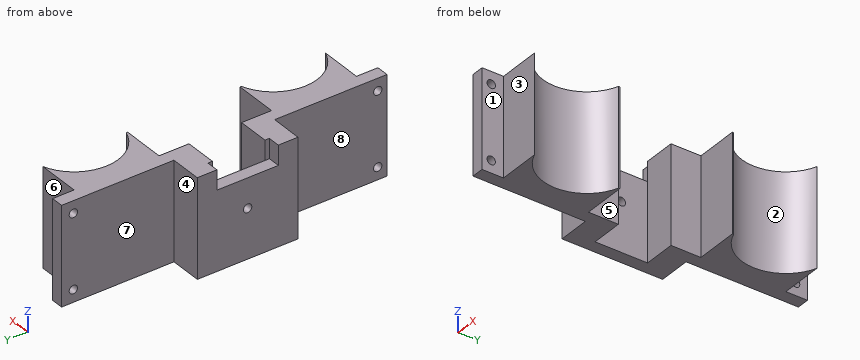
```python
from build123d import *

# Parameters (mm, degrees)
BOSS_EXTRUDE1_DEPTH  = 40
M3_CLEARANCE_HOLE1_D = 3.4
SKETCH6_W            = 5
SKETCH6_H            = 25
CUT_EXTRUDE1_DEPTH   = 8
M3_CLEARANCE_HOLE2_D = 3.4


with BuildPart() as part:
    # Sketch1 → Boss-Extrude1 (new body)
    with BuildSketch(Plane.XY):
        with BuildLine():
            Line((5, 0), (0, 0))
            Line((0, 0), (0, -20.5))
            Line((0, -20.5), (13, -20.5))
            Line((13, -20.5), (13, -66.25))
            Line((13, -66.25), (18, -66.25))
            Line((18, -66.25), (18, -57.5))
            Line((18, -57.5), (35.314368035, -57.5))
            ThreePointArc((35.314368035, -57.5), (23.250292021, -40.40428558), (35.508342613, -23.447116675))
            Line((35.508342613, -23.447116675), (35.508342613, -22.9))
            Line((35.508342613, -22.9), (18, -22.9))
            Line((18, -22.9), (18, -10.7))
            Line((18, -10.7), (5, -10.7))
            Line((5, -10.7), (5, 0))
        make_face()
    boss_extrude1 = extrude(amount=BOSS_EXTRUDE1_DEPTH)

    # Mirror1: Boss-Extrude1 across plane
    add(boss_extrude1.mirror(Plane.ZX))

    # M3 Clearance Hole1 (through all)
    with Locations(Plane.ZY.offset(-13)):
        with Locations((35, -62.481816862), (5, -62.481816862), (35, 61.468183138), (5, 61.468183138)):
            Hole(M3_CLEARANCE_HOLE1_D / 2)

    # Sketch6 → Cut-Extrude1 (cut)
    with BuildSketch(Plane(origin=(0, 0, 40), x_dir=(-1, 0, 0), z_dir=(0, 0, -1))):
        with Locations((-2.5, 0)):
            Rectangle(SKETCH6_W, SKETCH6_H)
    extrude(amount=CUT_EXTRUDE1_DEPTH, mode=Mode.SUBTRACT)

    # M3 Clearance Hole2 (through all)
    with Locations(Plane.ZY):
        with Locations((20, 0)):
            Hole(M3_CLEARANCE_HOLE2_D / 2)


solid = part.part
```
Can you work these out from the model? Positions are in its coordinate system, mm. Face numbers are marked on the shaded views. A direction names the side the tool comes from. Coordinates: 2 decimals unless noted, no trailing zeros. Loops run counter-clockwise (first coordinate to the right, second up) from the corner with the lowest first, then second, coordinate; pieces in that order, holes last. Notation, with made-up numbers: (-29, -3) - (-19, -3) arc R24 ccw to (-19, 31) - close; hole circle Ø2 at (4.5, 78). An arc over 180 degrees is marked (long way). Answer as CSV lines item,"result". Start each with the question number.
1) Thinking about a two-plate mould opening in Y: for the marked faces 1, 2, 3 and 4, which applies, pulls with the +Y half, pulls with the -Y half, needs draft (parallel to the pull), parting line crosses it, or undercut?
2) Suppose I cut it at C-C (x = 16). Please give me the cut outline in (y, z).
3) Which directions (+Z, -Z, +X, -X, +Y, -Y) give clear straight access to the entire face, cutting with the end or side of a thin tool? Please do the marked faces 5, 6, 7 and 8.
4) For pin 1 (1 mm diameter, centred on x = 30.5, z = 29.5, fed in from +Y); pin 2 (7 mm diameter, centred on y = -61.5, z = 19.5, fed in from +X); pin 3 (5 mm diameter, centred on y = 29.5, z = 11, fed in from +X), each with a flat end and sliding along its axis, tell me the tip position at first contact or that it passes through.
5) Suppose I cut it at A-A (z = 20). Please give me the cut outline in (x, y).
6) Suppose I cut it at B-B (y = 0). Please give me the cut outline in (x, z).
7) Suppose I cut it at D-D (z = 35). Count the separate pieces of the cut face and the enclosed holes in it, plus the area to 3 significant figures.
8) I need wall thicknesses on line 1 (Y direction, x = 15, z = 35); line 2 (Y direction, x = 19, z = 19); line 3 (Y direction, x = 31.5, z = 16). Which ranges of each line are inside material? Lowest first, please. Write a range as from..to.
Check result:
1,face 1,"needs draft"
1,face 2,"undercut"
1,face 3,"pulls with the -Y half"
1,face 4,"pulls with the +Y half"
2,outline,"(-66.25, 0) - (-10.7, 0) - (-10.7, 40) - (-66.25, 40) - close; (10.7, 0) - (66.25, 0) - (66.25, 40) - (10.7, 40) - close; hole circle Ø3.4 at (-62.48, 5); hole circle Ø3.4 at (-62.48, 35); hole circle Ø3.4 at (61.47, 5); hole circle Ø3.4 at (61.47, 35)"
3,face 5,"+Z, -Z, +X"
3,face 6,"+Z, -Z, +X, +Y"
3,face 7,"+Z, -Z, -X, +Y"
3,face 8,"+Z, -Z, -X, -Y"
4,pin 1,"stops at y = 57.5"
4,pin 2,"stops at x = 18"
4,pin 3,"stops at x = 29.35"
5,outline,"(0, -20.5) - (13, -20.5) - (13, -66.25) - (18, -66.25) - (18, -57.5) - (35.31, -57.5) arc R18 cw to (35.51, -23.45) - (35.51, -22.9) - (18, -22.9) - (18, -10.7) - (5, -10.7) - (5, -1.7) - (0, -1.7) - close; (0, 1.7) - (5, 1.7) - (5, 10.7) - (18, 10.7) - (18, 22.9) - (35.51, 22.9) - (35.51, 23.45) arc R18 cw to (35.31, 57.5) - (18, 57.5) - (18, 66.25) - (13, 66.25) - (13, 20.5) - (0, 20.5) - close"
6,outline,"(0, 0) - (5, 0) - (5, 18.3) - (0, 18.3) - close; (0, 21.7) - (5, 21.7) - (5, 32) - (0, 32) - close"
7,separate pieces,"4"
7,enclosed holes,"0"
7,area,"1,360 mm²"
8,line 1,"y = -66.25..-64.18, -60.78..-10.7, 10.7..59.77, 63.17..66.25"
8,line 2,"y = -57.5..-22.9, 22.9..57.5"
8,line 3,"y = -57.5..-55.64, -25.38..-22.9, 22.9..25.38, 55.64..57.5"
